The figure shows three views and two pictorial views of one solid part (mm, origin at its lowest corner). Answer the questions. A direction names the side the tool comes from. Round coordinates to 2 decimals unless told otherwise and drop trailing zeros. Order: outer loops, then holes, each group sorted by start corner. A loop starts at its lowest first (then second) coordinate and runs counter-clockwise, first axis right, second up. Notation, with made-up numbers: (89, 2.25) - (103, 2.25) arc R13 ccw to (103, 22.25) - close; hole circle Ø10 at (76, 68.5). An arc over 180 degrees is marked (long way). Use CSV: the item, a comma, the result in double quotes. Start each with the question number.
Item 1: Find section D-D, the plane z = 0.75. Give the vertices of the cut face in (x, y).
Item 2: Find section C-C, the plane x = 3.25. Give the vertices of the cut face in (y, z).
Item 3: Find section A-A, the plane z = 2.8. Give the vertices of the cut face in (x, y).
Item 4: Flat-ended cylindrical pins translate along their axes: P1, Ø2, axis at x = 3.5, y = 14, coming from the +Z side; P2, Ø0.6, axis at y = 19.5, z = 1, coming from the +X side. Find the tip coordinate at first contact, or state that the pin passes through.
Item 5: Find section B-B, the plane y = 24. Give the vertices of the cut face in (x, z), plus the area to 4 significant figures.
Item 6: Straight lines are drawn through the part: line 1 along Y through (x, z) = (2.5, 3.55); line 2 along Y through (x, z) = (3.5, 1.6); line 3 along X through (y, z) = (10.25, 0.6). For each, find the intervals that lie inside material, in ascending order. Write a range as [from, to].
Item 7: Determine the mould class of the marked faces 3, 4 and 5 for opening direction X: +X half, -X half, draft (parallel to the pull), parting line (faces both ways), or undercut.
Item 8: For the marked faces 1 and 2, determine the directions among +Z, -Z, +X, -X, +Y, -Y from which every point of the face is accessible in a straight line to the end or side of a thin tool.
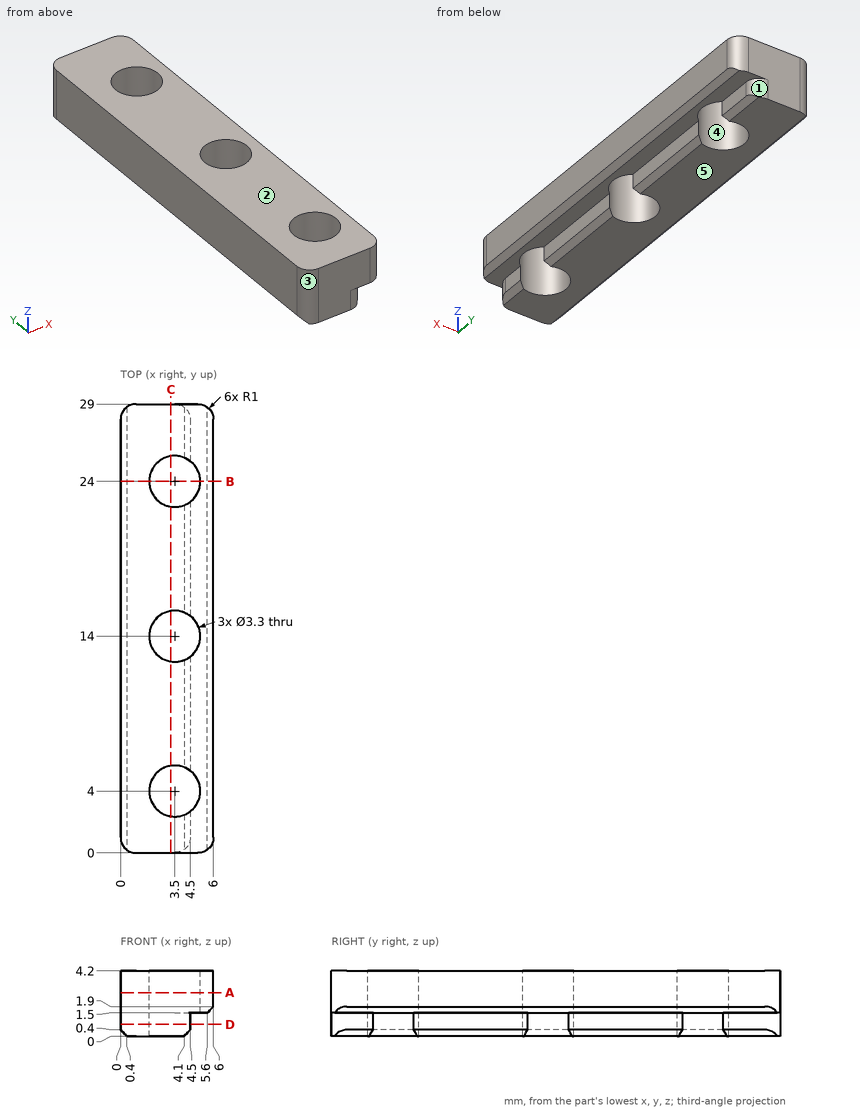
Worked out:
1,outline,"(0, 1) arc R1 ccw to (1, 0) - (3.5, 0) arc R1 ccw to (4.5, 1) - (4.5, 2.69) arc R1.65 cw (long way) to (4.5, 5.31) - (4.5, 12.69) arc R1.65 cw (long way) to (4.5, 15.31) - (4.5, 22.69) arc R1.65 cw (long way) to (4.5, 25.31) - (4.5, 28) arc R1 ccw to (3.5, 29) - (1, 29) arc R1 ccw to (0, 28) - close"
2,outline,"(0, 0) - (2.37, 0) - (2.37, 4.2) - (0, 4.2) - close; (5.63, 0) - (12.37, 0) - (12.37, 4.2) - (5.63, 4.2) - close; (15.63, 0) - (22.37, 0) - (22.37, 4.2) - (15.63, 4.2) - close; (25.63, 0) - (29, 0) - (29, 4.2) - (25.63, 4.2) - close"
3,outline,"(0, 1) arc R1 ccw to (1, 0) - (5, 0) arc R1 ccw to (6, 1) - (6, 28) arc R1 ccw to (5, 29) - (1, 29) arc R1 ccw to (0, 28) - close; hole circle Ø3.3 at (3.5, 4); hole circle Ø3.3 at (3.5, 14); hole circle Ø3.3 at (3.5, 24)"
4,P1,"passes through"
4,P2,"stops at x = 4.5"
5,outline,"(0, 0.4) - (0.4, 0) - (1.85, 0) - (1.85, 4.2) - (0, 4.2) - close; (5.15, 1.5) - (5.6, 1.5) - (6, 1.9) - (6, 4.2) - (5.15, 4.2) - close"
5,area,"9.905 mm²"
6,line 1,"y = [0, 2.69], [5.31, 12.69], [15.31, 22.69], [25.31, 29]"
6,line 2,"y = [0, 2.35], [5.65, 12.35], [15.65, 22.35], [25.65, 29]"
6,line 3,"x = [0, 4.5]"
7,face 3,"-X half"
7,face 4,"undercut"
7,face 5,"draft"
8,face 1,"-Z, +X, +Y"
8,face 2,"+Z, +X, -X, +Y, -Y"
